from build123d import *

# Parameters (mm, degrees)
SKETCH1_R                       = 20
SKETCH1_R_2                     = 1
BOSS_EXTRUDE1_DEPTH             = 22.5
TAP_DRILL_FOR_M5X0_8_TAP1_D     = 4.2
TAP_DRILL_FOR_M5X0_8_TAP1_DEPTH = 5
TAP_DRILL_FOR_M5X0_8_TAP1_TIP   = 1.2618073
SKETCH4_W                       = 2.794
SKETCH4_H                       = 6.604
CUT_EXTRUDE1_DEPTH              = 20.5
CIRPATTERN1_COUNT               = 5
CUT_EXTRUDE3_START              = -6
SKETCH6_W                       = 4.62
SKETCH6_H                       = 8
SKETCH6_R                       = 2.1
CUT_EXTRUDE3_DEPTH              = 6
SKETCH7_R                       = 5.5
CUT_EXTRUDE4_DEPTH              = 1.8
SKETCH9_R                       = 3.014010562
CUT_EXTRUDE5_DEPTH              = 2
CHAMFER1_SIZE                   = 2
SKETCH8_R                       = 20
SKETCH8_R_2                     = 3
BOSS_EXTRUDE2_DEPTH             = 3
SKETCH5_R                       = 6
SKETCH5_R_2                     = 5
CUT_EXTRUDE2_DEPTH              = 1
FILLET3_R                       = 0.5
FILLET4_R                       = 2
SKETCH10_W                      = 43.83789535
SKETCH10_H                      = 47.8950696
CUT_EXTRUDE6_DEPTH              = 16


with BuildPart() as part:
    # Sketch1 → Boss-Extrude1 (new body)
    with BuildSketch(Plane.XY):
        with Locations(Location((-11.822558412, 14.529752947, 0), (0, 0, 180))):
            Circle(SKETCH1_R)
        with Locations(Location((-11.822558412, 14.529752947, 0), (0, 0, 180))):
            Circle(SKETCH1_R_2, mode=Mode.SUBTRACT)
    extrude(amount=BOSS_EXTRUDE1_DEPTH)

    # Tap Drill for M5x0.8 Tap1
    with Locations(Plane.XY.offset(22.5)):
        with Locations((-11.822558412, 14.529752947)):
            Hole(TAP_DRILL_FOR_M5X0_8_TAP1_D / 2, depth=TAP_DRILL_FOR_M5X0_8_TAP1_DEPTH)
            with Locations((0, 0, -(TAP_DRILL_FOR_M5X0_8_TAP1_DEPTH + TAP_DRILL_FOR_M5X0_8_TAP1_TIP / 2))):  # 118° drill point
                Cone(0, TAP_DRILL_FOR_M5X0_8_TAP1_D / 2, TAP_DRILL_FOR_M5X0_8_TAP1_TIP, mode=Mode.SUBTRACT)

    # Sketch4 → Cut-Extrude1 (cut)
    with BuildSketch(Plane.XY.offset(22.5)):
        with Locations((4.780441588, 14.531752947)):
            Rectangle(SKETCH4_W, SKETCH4_H)
    cut_extrude1 = extrude(amount=-CUT_EXTRUDE1_DEPTH, mode=Mode.SUBTRACT)

    # CirPattern1: Cut-Extrude1 ×5 about axis
    cirpattern1_axis = Axis((-11.822558412, 14.529752947, 0), (0, 0, 1))
    for i in range(1, CIRPATTERN1_COUNT):
        add(cut_extrude1.rotate(cirpattern1_axis, i * 360 / CIRPATTERN1_COUNT), mode=Mode.SUBTRACT)

    # Sketch6 → Cut-Extrude3 (cut)
    # profile 1 of 4: a face of its own
    with BuildSketch(Plane.XY.offset(22.5).offset(CUT_EXTRUDE3_START)):
        Polygon((-16.444354251, 14.529752947), (-14.132558412, 18.529752947), (-14.132558412, 10.529752947), align=None)
    # profile 2 of 4: a face of its own
    with BuildSketch(Plane.XY.offset(22.5).offset(CUT_EXTRUDE3_START)):
        Polygon((-7.200762573, 14.529752947), (-9.512558412, 10.529752947), (-9.512558412, 18.529752947), align=None)
    # profile 3 of 4: a face of its own
    with BuildSketch(Plane.XY.offset(22.5).offset(CUT_EXTRUDE3_START)):
        with Locations((-11.822558412, 14.529752947)):
            Rectangle(SKETCH6_W, SKETCH6_H)
        with Locations((-11.822558412, 14.529752947)):
            Circle(SKETCH6_R, mode=Mode.SUBTRACT)
    # profile 4 of 4: a face of its own
    with BuildSketch(Plane.XY.offset(22.5).offset(CUT_EXTRUDE3_START)):
        with Locations((-11.822558412, 14.529752947)):
            Circle(SKETCH6_R)
    extrude(amount=CUT_EXTRUDE3_DEPTH, mode=Mode.SUBTRACT)

    # Sketch7 → Cut-Extrude4 (cut)
    with BuildSketch(Plane.XY.offset(22.5)):
        with Locations((-11.822558412, 14.529752947)):
            Circle(SKETCH7_R)
    extrude(amount=-CUT_EXTRUDE4_DEPTH, mode=Mode.SUBTRACT)

    # Sketch9 → Cut-Extrude5 (cut)
    with BuildSketch(Plane.XY.offset(16.5)):
        with Locations((-11.822558412, 14.529752947)):
            Circle(SKETCH9_R)
    extrude(amount=-CUT_EXTRUDE5_DEPTH, mode=Mode.SUBTRACT)

    # Chamfer1
    chamfer1_edges = [part.edges().sort_by_distance(p)[0] for p in [
        (-14.836568974, 14.529752947, 14.5),
    ]]
    chamfer(chamfer1_edges, length=CHAMFER1_SIZE - 0.0001)  # a hair under: the kernel refuses the full size

    # Sketch8 → Boss-Extrude2 (add)
    with BuildSketch(Plane.XY.offset(22.5)):
        with Locations(Location((-11.822558412, 14.529752947, 0), (0, 0, 180))):
            Circle(SKETCH8_R)
        with Locations((-11.822558412, 14.529752947)):
            Circle(SKETCH8_R_2, mode=Mode.SUBTRACT)
    extrude(amount=BOSS_EXTRUDE2_DEPTH)

    # Sketch5 → Cut-Extrude2 (cut)
    with BuildSketch(Plane(origin=(0, 0, 0), x_dir=(-1, 0, 0), z_dir=(0, 0, -1))):
        with Locations((11.822558412, 14.529752947)):
            Circle(SKETCH5_R)
        with Locations((11.822558412, 14.529752947)):
            Circle(SKETCH5_R_2, mode=Mode.SUBTRACT)
    extrude(amount=-CUT_EXTRUDE2_DEPTH, mode=Mode.SUBTRACT)

    # Fillet3
    fillet3_edges = [part.edges().sort_by_distance(p)[0] for p in [
        (-5.822558412, 14.529752947, 1),
        (-6.822558412, 14.529752947, 1),
    ]]
    fillet(fillet3_edges, radius=FILLET3_R - 0.0001)  # a hair under: the kernel refuses the full size

    # Fillet4
    fillet4_edges = [part.edges().sort_by_distance(p)[0] for p in [
        (8.177441588, 14.529752947, 25.5),
    ]]
    fillet(fillet4_edges, radius=FILLET4_R)

    # Sketch10 → Cut-Extrude6 (cut)
    with BuildSketch(Plane(origin=(0, 0, 0), x_dir=(-1, 0, 0), z_dir=(0, 0, -1))):
        with Locations((12.103243423, 14.057691792)):
            Rectangle(SKETCH10_W, SKETCH10_H)
    extrude(amount=-CUT_EXTRUDE6_DEPTH, mode=Mode.SUBTRACT)


solid = part.part
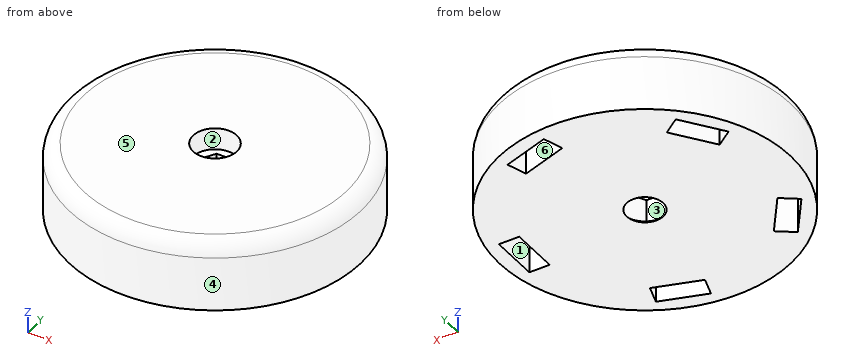
Model file for the job. Use its own axes, mm. Face numbers are marked on the shaded views. A direction names the side the tool comes from. Coordinates: 2 decimals unless noted, no trailing zeros. Order: outer loops, then holes, each group sorted by start corner. A loop starts at its lowest first (then second) coordinate and runs counter-clockwise, first axis right, second up. Notation, with made-up numbers: M -13.5,66 L 13.5,66 A18 cw 13.5,87 Z; hole C 26.25,4.25 d4. An arc over 180 degrees is marked long. Return JSON: item names as keys, results as strings.
1. Saw through at A-A (z = 19.5). Give the cut face in (x, y), and give its area (3 significant figures).
Ans:
{"outline": "C -11.82,14.53 d40; hole M -28.33,22.44 L -26.07,20.79 L -22.18,26.14 L -24.45,27.78 Z; hole M -28.32,6.62 L -24.44,1.28 L -22.18,2.92 L -26.06,8.26 Z; hole M -16.44,14.53 L -14.13,10.53 L -9.51,10.53 L -7.2,14.53 L -9.51,18.53 L -14.13,18.53 Z; hole M -10.27,30.01 L -3.99,27.97 L -3.12,30.63 L -9.4,32.67 Z; hole M -10.26,-0.95 L -9.4,-3.61 L -3.12,-1.57 L -3.98,1.09 Z; hole M 3.38,11.23 L 6.18,11.23 L 6.18,17.83 L 3.38,17.83 Z", "area": "1,110 mm^2"}
2. Flat gauge pins, fed straight in: pin 1 (2 mm diameter, centred on x = 5, y = 16, fed in from -Z); pin 2 (3 mm diameter, centred on x = 4.5, z = 19.5, fed in from +Y); pin 3 (5 mm diameter, centred on y = 29.5, z = 22, fed in from +X). Where does each tip first touch, or does it go through?
Ans:
{"pin 1": "z = 22.5", "pin 2": "y = 27.96", "pin 3": "x = 3.81"}
3. Tool access for the marked faces 1, 2 and 3: list every direction of +Z, -Z, +X, -X, +Y, -Y with a clear straight run to the whole face (end or side of a thin tool).
Ans:
{"face 1": "-Z", "face 2": "+Z", "face 3": "none"}
4. Pull direction X, two halves, no side cores. Call the marked faces 4, 5 and 6: +X half, -X half, draft (parallel to the pull), parting line (faces both ways), or undercut.
Ans:
{"face 4": "parting line", "face 5": "draft", "face 6": "undercut"}
5. Saw through at B-B (z = 23). Give the cut face in (x, y).
Ans:
{"outline": "C -11.82,14.53 d40; hole C -11.82,14.53 d6"}
6. Drill centre lines: probe 1 along Y at (x, z) = (-8.5, 18.75); probe 2 along Y at (x, z) = (-26, 17); probe 3 along Y at (x, z) = (-9, 17). Where is each one in solid material? Low to high.
Ans:
{"probe 1": "-5.19 to -3.32, -0.38 to 12.28, 16.78 to 29.44, 32.38 to 34.25", "probe 2": "0.42 to 3.42, 8.17 to 20.89, 25.64 to 28.64", "probe 3": "-5.27 to -3.48, -0.54 to 11.42, 17.64 to 29.6, 32.54 to 34.33"}
